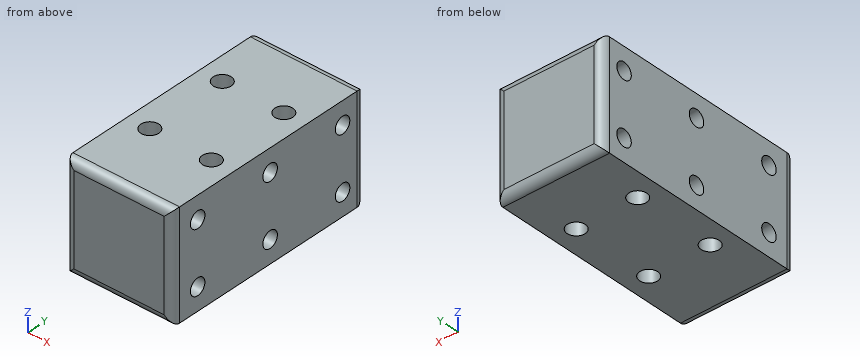
```python
from build123d import *

# Parameters (mm, degrees)
SKETCH_1_W          = 26
SKETCH_1_H          = 26
EXTRUDE_1_DEPTH     = 53
FILLET_2_R          = 2
CUT_EXTRUDE_1_REACH = 62.448
SKETCH_2_R          = 1.55
CUT_EXTRUDE_2_REACH = 62.448
SKETCH_3_R          = 2
CUT_EXTRUDE_3_REACH = 62.448
SKETCH_4_R          = 2.2


with BuildPart() as part:
    # 草图1 → 凸台-拉伸1 (new body)
    with BuildSketch(Plane(origin=(0, 0, 0), x_dir=(1, 0, 0), z_dir=(0, 1, 0))):
        Rectangle(SKETCH_1_W, SKETCH_1_H)
    extrude(amount=EXTRUDE_1_DEPTH)

    # 圆角2
    fillet_2_edges = [part.edges().sort_by_distance(p)[0] for p in [
        (-13, 53, 0),
        (0, 53, 13),
        (13, 53, 0),
        (0, 0, 13),
        (-13, 0, 0),
        (0, 0, -13),
        (13, 0, 0),
        (0, 53, -13),
    ]]
    fillet(fillet_2_edges, radius=FILLET_2_R)

    # 草图2 → 切除-拉伸1 (cut, up to next)
    with BuildSketch(Plane.XY.offset(13), mode=Mode.PRIVATE) as cut_extrude_1_sk1:
        with Locations((-7.5, 37)):
            Circle(SKETCH_2_R)
    cut_extrude_1_tool1 = extrude(cut_extrude_1_sk1.sketch, amount=-CUT_EXTRUDE_1_REACH, mode=Mode.PRIVATE) & part.part
    # 草图2 → 切除-拉伸1 (cut, up to next)
    with BuildSketch(Plane.XY.offset(13), mode=Mode.PRIVATE) as cut_extrude_1_sk2:
        with Locations((7.5, 37)):
            Circle(SKETCH_2_R)
    cut_extrude_1_tool2 = extrude(cut_extrude_1_sk2.sketch, amount=-CUT_EXTRUDE_1_REACH, mode=Mode.PRIVATE) & part.part
    # 草图2 → 切除-拉伸1 (cut, up to next)
    with BuildSketch(Plane.XY.offset(13), mode=Mode.PRIVATE) as cut_extrude_1_sk3:
        with Locations((-7.5, 17)):
            Circle(SKETCH_2_R)
    cut_extrude_1_tool3 = extrude(cut_extrude_1_sk3.sketch, amount=-CUT_EXTRUDE_1_REACH, mode=Mode.PRIVATE) & part.part
    # 草图2 → 切除-拉伸1 (cut, up to next)
    with BuildSketch(Plane.XY.offset(13), mode=Mode.PRIVATE) as cut_extrude_1_sk4:
        with Locations((7.5, 17)):
            Circle(SKETCH_2_R)
    cut_extrude_1_tool4 = extrude(cut_extrude_1_sk4.sketch, amount=-CUT_EXTRUDE_1_REACH, mode=Mode.PRIVATE) & part.part
    add(cut_extrude_1_tool1.solids().sort_by_distance((-7.5, 37, 13))[0], mode=Mode.SUBTRACT)
    add(cut_extrude_1_tool2.solids().sort_by_distance((7.5, 37, 13))[0], mode=Mode.SUBTRACT)
    add(cut_extrude_1_tool3.solids().sort_by_distance((-7.5, 17, 13))[0], mode=Mode.SUBTRACT)
    add(cut_extrude_1_tool4.solids().sort_by_distance((7.5, 17, 13))[0], mode=Mode.SUBTRACT)

    # 草图3 → 切除-拉伸2 (cut, up to next)
    with BuildSketch(Plane.ZY.offset(13), mode=Mode.PRIVATE) as cut_extrude_2_sk1:
        with Locations((-7.5, 47)):
            Circle(SKETCH_3_R)
    cut_extrude_2_tool1 = extrude(cut_extrude_2_sk1.sketch, amount=-CUT_EXTRUDE_2_REACH, mode=Mode.PRIVATE) & part.part
    # 草图3 → 切除-拉伸2 (cut, up to next)
    with BuildSketch(Plane.ZY.offset(13), mode=Mode.PRIVATE) as cut_extrude_2_sk2:
        with Locations((7.5, 47)):
            Circle(SKETCH_3_R)
    cut_extrude_2_tool2 = extrude(cut_extrude_2_sk2.sketch, amount=-CUT_EXTRUDE_2_REACH, mode=Mode.PRIVATE) & part.part
    # 草图3 → 切除-拉伸2 (cut, up to next)
    with BuildSketch(Plane.ZY.offset(13), mode=Mode.PRIVATE) as cut_extrude_2_sk3:
        with Locations((-7.5, 27)):
            Circle(SKETCH_3_R)
    cut_extrude_2_tool3 = extrude(cut_extrude_2_sk3.sketch, amount=-CUT_EXTRUDE_2_REACH, mode=Mode.PRIVATE) & part.part
    # 草图3 → 切除-拉伸2 (cut, up to next)
    with BuildSketch(Plane.ZY.offset(13), mode=Mode.PRIVATE) as cut_extrude_2_sk4:
        with Locations((7.5, 27)):
            Circle(SKETCH_3_R)
    cut_extrude_2_tool4 = extrude(cut_extrude_2_sk4.sketch, amount=-CUT_EXTRUDE_2_REACH, mode=Mode.PRIVATE) & part.part
    # 草图3 → 切除-拉伸2 (cut, up to next)
    with BuildSketch(Plane.ZY.offset(13), mode=Mode.PRIVATE) as cut_extrude_2_sk5:
        with Locations((-7.5, 7)):
            Circle(SKETCH_3_R)
    cut_extrude_2_tool5 = extrude(cut_extrude_2_sk5.sketch, amount=-CUT_EXTRUDE_2_REACH, mode=Mode.PRIVATE) & part.part
    # 草图3 → 切除-拉伸2 (cut, up to next)
    with BuildSketch(Plane.ZY.offset(13), mode=Mode.PRIVATE) as cut_extrude_2_sk6:
        with Locations((7.5, 7)):
            Circle(SKETCH_3_R)
    cut_extrude_2_tool6 = extrude(cut_extrude_2_sk6.sketch, amount=-CUT_EXTRUDE_2_REACH, mode=Mode.PRIVATE) & part.part
    add(cut_extrude_2_tool1.solids().sort_by_distance((-13, 47, -7.5))[0], mode=Mode.SUBTRACT)
    add(cut_extrude_2_tool2.solids().sort_by_distance((-13, 47, 7.5))[0], mode=Mode.SUBTRACT)
    add(cut_extrude_2_tool3.solids().sort_by_distance((-13, 27, -7.5))[0], mode=Mode.SUBTRACT)
    add(cut_extrude_2_tool4.solids().sort_by_distance((-13, 27, 7.5))[0], mode=Mode.SUBTRACT)
    add(cut_extrude_2_tool5.solids().sort_by_distance((-13, 7, -7.5))[0], mode=Mode.SUBTRACT)
    add(cut_extrude_2_tool6.solids().sort_by_distance((-13, 7, 7.5))[0], mode=Mode.SUBTRACT)

    # 草图4 → 切除-拉伸3 (cut, up to next)
    with BuildSketch(Plane(origin=(0, 0, -13), x_dir=(-1, 0, 0), z_dir=(0, 0, -1)), mode=Mode.PRIVATE) as cut_extrude_3_sk1:
        with Locations((-7.5, 37)):
            Circle(SKETCH_4_R)
    cut_extrude_3_tool1 = extrude(cut_extrude_3_sk1.sketch, amount=-CUT_EXTRUDE_3_REACH, mode=Mode.PRIVATE) & part.part
    # 草图4 → 切除-拉伸3 (cut, up to next)
    with BuildSketch(Plane(origin=(0, 0, -13), x_dir=(-1, 0, 0), z_dir=(0, 0, -1)), mode=Mode.PRIVATE) as cut_extrude_3_sk2:
        with Locations((7.5, 37)):
            Circle(SKETCH_4_R)
    cut_extrude_3_tool2 = extrude(cut_extrude_3_sk2.sketch, amount=-CUT_EXTRUDE_3_REACH, mode=Mode.PRIVATE) & part.part
    # 草图4 → 切除-拉伸3 (cut, up to next)
    with BuildSketch(Plane(origin=(0, 0, -13), x_dir=(-1, 0, 0), z_dir=(0, 0, -1)), mode=Mode.PRIVATE) as cut_extrude_3_sk3:
        with Locations((7.5, 17)):
            Circle(SKETCH_4_R)
    cut_extrude_3_tool3 = extrude(cut_extrude_3_sk3.sketch, amount=-CUT_EXTRUDE_3_REACH, mode=Mode.PRIVATE) & part.part
    # 草图4 → 切除-拉伸3 (cut, up to next)
    with BuildSketch(Plane(origin=(0, 0, -13), x_dir=(-1, 0, 0), z_dir=(0, 0, -1)), mode=Mode.PRIVATE) as cut_extrude_3_sk4:
        with Locations((-7.5, 17)):
            Circle(SKETCH_4_R)
    cut_extrude_3_tool4 = extrude(cut_extrude_3_sk4.sketch, amount=-CUT_EXTRUDE_3_REACH, mode=Mode.PRIVATE) & part.part
    add(cut_extrude_3_tool1.solids().sort_by_distance((7.5, 37, -13))[0], mode=Mode.SUBTRACT)
    add(cut_extrude_3_tool2.solids().sort_by_distance((-7.5, 37, -13))[0], mode=Mode.SUBTRACT)
    add(cut_extrude_3_tool3.solids().sort_by_distance((-7.5, 17, -13))[0], mode=Mode.SUBTRACT)
    add(cut_extrude_3_tool4.solids().sort_by_distance((7.5, 17, -13))[0], mode=Mode.SUBTRACT)


solid = part.part
```
Read the model definition and answer for the solid it produces. Units are mm, in the model's axes. Give positions to 0.01 mm unless a question says otherwise; leave off trailing zeros. Write each loop counter-clockwise with the first axis right and the second up, starting at its lowest first coordinate (ties: lowest second). Pieces come first, ordered by that corner, then holes. Notation, with made-up numbers: (18, -2) -> (43, -2) arc R31 ccw to (43, 27) -> close; hole circle Ø5 at (-15.5, 6). An arc over 180 degrees is marked (long way). Answer in a Markdown table with one row per item.
1) Section C-C on x = -7.5 is taken. Count the separate pieces of the cut face and the enclosed holes in it, plus the area to 3 significant figures.
Results list:
| item | result |
|---|---|
| separate pieces | 3 |
| enclosed holes | 6 |
| area | 1,070 mm^2 |
2) Section A-A on z = 7.5 is taken. Give the vertices of the cut face in (x, y).
Results list:
| item | result |
|---|---|
| outline | (-13, 2) arc R2 ccw to (-11, 0) -> (11, 0) arc R2 ccw to (13, 2) -> (13, 5) -> (-13, 5) -> close; (-13, 9) -> (13, 9) -> (13, 25) -> (-13, 25) -> close; (-13, 29) -> (13, 29) -> (13, 45) -> (-13, 45) -> close; (-13, 49) -> (13, 49) -> (13, 51) arc R2 ccw to (11, 53) -> (-11, 53) arc R2 ccw to (-13, 51) -> close; hole circle Ø4.4 at (-7.5, 17); hole circle Ø4.4 at (-7.5, 37); hole circle Ø4.4 at (7.5, 17); hole circle Ø4.4 at (7.5, 37) |
3) Section D-D on z = -1 is taken. Give the vertices of the cut face in (x, y), plus the area to 3 significant figures.
Results list:
| item | result |
|---|---|
| outline | (-13, 2) arc R2 ccw to (-11, 0) -> (11, 0) arc R2 ccw to (13, 2) -> (13, 51) arc R2 ccw to (11, 53) -> (-11, 53) arc R2 ccw to (-13, 51) -> close; hole circle Ø4.4 at (-7.5, 17); hole circle Ø4.4 at (-7.5, 37); hole circle Ø4.4 at (7.5, 17); hole circle Ø4.4 at (7.5, 37) |
| area | 1,310 mm^2 |
4) Section B-B on y = 47 is taken. Give the vertices of the cut face in (x, z), plus the area to 3 significant figures.
Results list:
| item | result |
|---|---|
| outline | (-13, -13) -> (13, -13) -> (13, -9.5) -> (-13, -9.5) -> close; (-13, -5.5) -> (13, -5.5) -> (13, 5.5) -> (-13, 5.5) -> close; (-13, 9.5) -> (13, 9.5) -> (13, 13) -> (-13, 13) -> close |
| area | 468 mm^2 |
5) Each of these flat-tipped pins is pushed along its axis until it touches: pin 1 Ø4 at (x, y) = (-7.5, 17) entering from +Z; pin 2 Ø5.5 at (x, y) = (7.5, 37) entering from +Z. Where does it stop, or does it pass through?
Results list:
| item | result |
|---|---|
| pin 1 | through |
| pin 2 | z = 13 |
6) Straight lines are drawn through the part: line 1 (Y direction, x = -0.25, z = 7.25); line 2 (Y direction, x = -5.5, z = 7.75); line 3 (X direction, y = 35, z = 4.25). For each, find the intervals that lie inside material, in ascending order. Write a range as [from, to].
Results list:
| item | result |
|---|---|
| line 1 | [0, 5.02], [8.98, 25.02], [28.98, 45.02], [48.98, 53] |
| line 2 | [0, 5.02], [8.98, 16.08], [17.92, 25.02], [28.98, 36.08], [37.92, 45.02], [48.98, 53] |
| line 3 | [-13, -8.42], [-6.58, 6.58], [8.42, 13] |
